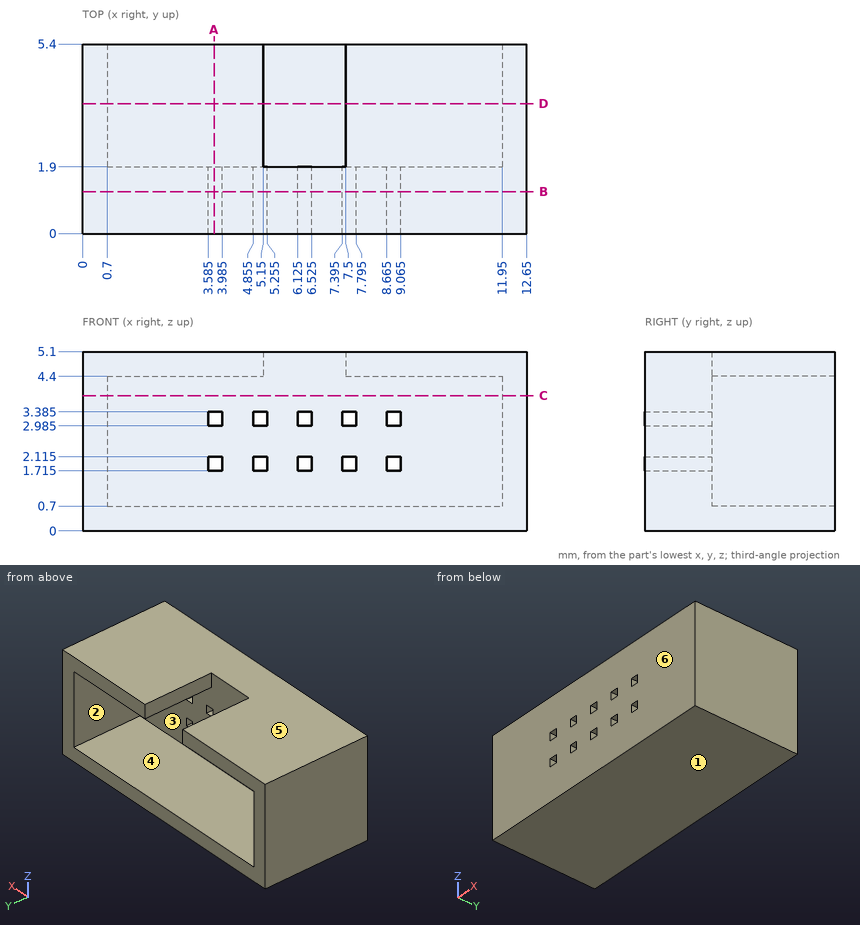
Source: three-view drawing plus pictorial views. Frame: mm from the lowest corner of the part. A direction names the side the tool comes from. Coordinates: 2 decimals unless noted, no trailing zeros. Order: outer loops, then holes, each group sorted by start corner. A loop starts at its lowest first (then second) coordinate and runs counter-clockwise, first axis right, second up. Notation, with made-up numbers: M 61.5,62.25 L 101.5,62.25 A11 cw 101.5,78.25 Z; hole C 83,69.25 d3. An arc over 180 degrees is marked long. One line per question, with ' | ' between items.
Item 1: Reachability of the marked faces 1 and 2 from +Z, -Z, +X, -X, +Y, -Y: full face, straight path, thin tool, end or side. Return the list, or none.
Geometry results:
face 1: -Z, +X, -X, +Y, -Y | face 2: +Y
Item 2: Ray query, line 1 along X through (y, z) = (2.4, 4.3); line 2 along Z through (x, y) = (10.5, 4.55); line 3 along X through (y, z) = (1.7, 3.3) (3 decimals). Return the intervals inside material, ascending.
Geometry results:
line 1: x = 0 to 0.7, 11.95 to 12.65 | line 2: z = 0 to 0.7, 4.4 to 5.1 | line 3: x = 0 to 3.585, 3.985 to 4.855, 5.255 to 6.125, 6.525 to 7.395, 7.795 to 8.665, 9.065 to 12.65
Item 3: Section C-C (z = 3.85). Output: boundary loops of the cut face in (x, y), then the cut area to 3 significant figures.
Geometry results:
outline: M 0,0 L 12.65,0 L 12.65,5.4 L 11.95,5.4 L 11.95,1.9 L 0.7,1.9 L 0.7,5.4 L 0,5.4 Z | area: 28.9 mm^2
Item 4: Section D-D (y = 3.7). Output: boundary loops of the cut face in (x, z), then the cut area to 3 significant figures.
Geometry results:
outline: M 0,0 L 12.65,0 L 12.65,5.1 L 7.5,5.1 L 7.5,4.4 L 11.95,4.4 L 11.95,0.7 L 0.7,0.7 L 0.7,4.4 L 5.15,4.4 L 5.15,5.1 L 0,5.1 Z | area: 21.2 mm^2
Item 5: Section A-A (x = 3.75). Output: boundary loops of the cut face in (y, z) (3 decimals).
Geometry results:
outline: M 0,0 L 5.4,0 L 5.4,0.7 L 1.9,0.7 L 1.9,1.715 L 0,1.715 Z; M 0,2.115 L 1.9,2.115 L 1.9,2.985 L 0,2.985 Z; M 0,3.385 L 1.9,3.385 L 1.9,4.4 L 5.4,4.4 L 5.4,5.1 L 0,5.1 Z
Item 6: Section B-B (y = 1.2). Give the number of separate pieces and of enclosed holes in the cut face, then the cut area to 3 significant figures.
Geometry results:
separate pieces: 1 | enclosed holes: 10 | area: 62.9 mm^2
Item 7: Draft query along Z for the marked faces 3, 4, 5 and 6. Return one class per face: released by +Z, released by -Z, zero draft, split by the parting line, or undercut.
Geometry results:
face 3: undercut | face 4: undercut | face 5: released by +Z | face 6: zero draft
Item 8: Pin query (flat end, axial travel): pin 1 (1 mm diameter, centred on x = 3.5, y = 3.5, fed in from -Z); pin 2 (1 mm diameter, centred on x = 7.5, z = 1.5, fed in from +Y). Return the tip coordinate at first contact, or that it passes through.
Geometry results:
pin 1: stops at z = 0 | pin 2: stops at y = 1.9
